Read the model definition and answer for the solid it produces. Units are mm, in the model's axes. A direction names the side the tool comes from. Coordinates: 2 decimals unless noted, no trailing zeros. Loops run counter-clockwise (first coordinate to the right, second up) from the corner with the lowest first, then second, coordinate; pieces in that order, holes last. Notation, with made-up numbers: M -34.75,-32 L -11.75,-32 A20 cw -11.75,-23 Z; hole C 37.5,-16.5 d10. An arc over 180 degrees is marked long. One line per item, written item: value. Start each with the question number.
1. Flat-ended cylindrical pins translate along their axes: pin 1 (15 mm diameter, centred on x = 52, z = 40, fed in from -Y); pin 2 (6 mm diameter, centred on x = 92.5, y = -17.5, fed in from -Z); pin 3 (8 mm diameter, centred on x = 57, z = 69.5, fed in from -Y); pin 4 (3 mm diameter, centred on x = 95.5, z = 4, fed in from -Y). Find the tip coordinate at first contact, or state that the pin passes through.
2. Consider probe 1 along X at (y, z) = (12.5, -2.5) (3 decimals); probe 2 along Y at (x, z) = (59, 47.5); probe 3 along Z at (x, y) = (17, 52) (3 decimals). Determine where each line is inside the solid, lowest interval first.
3. The part is cut by section A-A (y = -46). Write down the section's boundary in (x, z) (3 decimals), then the cut area to 3 significant figures.
4. The part is cut by section B-B (z = 110). Write down the section's boundary in (x, y).
5. For faces 1 (the face through (-2, 8.001, 31)), 2 (the face through (60, 0, 61.925)), 3 (the face through (109.2, -9.7, 52.6)), 4 (the face through (101, 10, 38.1)), determine the directions among +Z, -Z, +X, -X, +Y, -Y from which every point of the face is accessible in a straight line to the end or side of a thin tool.
```python
from build123d import *

# Parameters (mm, degrees)
F2_DEPTH     = 63.5
F0_W         = 25.4
F0_H         = 19.05
F3_DEPTH     = 25.4
F4_DEPTH     = 8.001
F6_R         = 6.35
F7_T1_DEPTH  = 17.4752
F7_T4_ANGLE  = 90
F7_T8_DEPTH  = 42.06875
F7_S9_R      = 25.4
F7_T10_DEPTH = 23
F7_T12_ANGLE = 90
F7_T14_ANGLE = 90
F7_T18_DEPTH = 42.06875
F7_S19_R     = 25.4
F7_T20_DEPTH = 23
F7_T22_ANGLE = 90
F7_T26_DEPTH = 42.06875
F7_S27_R     = 25.4
F7_T28_DEPTH = 23
F7_T32_DEPTH = 42.06875
F7_S33_R     = 25.4
F7_T34_DEPTH = 23
F8_R         = 19.05
F9_DEPTH     = 127


# Not quite as in the source:
# - a fillet or chamfer that OpenCascade refuses, or shapes differently, is made with other operations: its cross-section is extruded or revolved along the edge and cut away or added


with BuildPart() as f2:
    # F0 (on Front) → F2 (new body, symmetric)
    with BuildSketch(Plane.XZ):
        Polygon((22.225, 9.525), (-41.275, 9.525), (-41.275, -9.525), (41.275, -9.525), (41.275, 9.525), align=None)
    extrude(amount=F2_DEPTH, both=True)

    # F0 (on Front) → F3 (join, symmetric)
    with BuildSketch(Plane.XZ):
        with BuildLine():
            Line((22.225, 27.0002), (22.225, 9.525))
            Line((22.225, 9.525), (41.275, 9.525))
            Line((41.275, 9.525), (41.275, 27.0002))
            ThreePointArc((41.275, 27.0002), (45.9246798487, 38.2255201513), (57.15, 42.8752))
            Line((57.15, 42.8752), (60.325, 42.8752))
            Line((60.325, 42.8752), (60.325, 61.9252))
            Line((60.325, 61.9252), (57.15, 61.9252))
            ThreePointArc((57.15, 61.9252), (32.4542956671, 51.6959043329), (22.225, 27.0002))
        make_face()
        with Locations((73.025, 52.4002)):
            Rectangle(F0_W, F0_H)
    extrude(amount=F3_DEPTH, both=True)

    # F0 (on Front) → F4 (join, symmetric)
    with BuildSketch(Plane.XZ):
        with BuildLine():
            add(Edge.make_bspline(
                [(-41.275, 9.525), (-25.3429859877, 49.4523830712), (4.4616423547, 62.58662045), (57.15, 61.9252)],
                knots=[0, 0, 0, 0, 111.5045361635, 111.5045361635, 111.5045361635, 111.5045361635], degree=3))
            Line((-41.275, 9.525), (22.225, 9.525))
            Line((22.225, 9.525), (22.225, 27.0002))
            ThreePointArc((22.225, 27.0002), (32.4542956671, 51.6959043329), (57.15, 61.9252))
        make_face()
    extrude(amount=F4_DEPTH, both=True)

    # F0 (on Front) → F5 (revolve)
    with BuildSketch(Plane.XZ):
        Polygon((85.725, 66.675), (85.725, 61.9252), (85.725, 42.8752), (85.725, 38.1), (111.125, 38.1), (111.125, 66.675), align=None)
    revolve(axis=Axis((85.725, 0, 52.3875), (0, 0, 1)))

    # F6
    f6_edges = [f2.edges().sort_by_distance(p)[0] for p in [
        (41.275, -63.5, 0),
        (-41.275, -63.5, 0),
        (41.275, 63.5, 0),
        (-41.275, 63.5, 0),
    ]]
    fillet(f6_edges, radius=F6_R)

    # F7: fillet of radius 3.175 on 12 edges, made by hand

    # F7_s2 → F7_t1 (cut)
    with BuildSketch(Plane.XY.offset(9.525)):
        with BuildLine():
            ThreePointArc((25.4, -25.4), (23.1549359697, -24.4700640303), (22.225, -22.225))
            Line((22.225, -22.225), (22.225, -25.4))
            Line((22.225, -25.4), (25.4, -25.4))
        make_face()
        with BuildLine():
            ThreePointArc((41.275, -22.225), (40.3450640303, -24.4700640303), (38.1, -25.4))
            Line((38.1, -25.4), (41.275, -25.4))
            Line((41.275, -25.4), (41.275, -22.225))
        make_face()
        with BuildLine():
            ThreePointArc((25.4, 25.4), (23.1549359697, 24.4700640303), (22.225, 22.225))
            Line((22.225, 22.225), (22.225, 25.4))
            Line((22.225, 25.4), (25.4, 25.4))
        make_face()
        with BuildLine():
            ThreePointArc((41.275, 22.225), (40.3450640303, 24.4700640303), (38.1, 25.4))
            Line((38.1, 25.4), (41.275, 25.4))
            Line((41.275, 25.4), (41.275, 22.225))
        make_face()
    extrude(amount=F7_T1_DEPTH, mode=Mode.SUBTRACT)

    # F7_s3 → F7_t4 (revolve, cut)
    with BuildSketch(Plane.YZ.offset(57.15)):
        with BuildLine():
            ThreePointArc((-25.4, 58.7502), (-24.4700640303, 60.9952640303), (-22.225, 61.9252))
            Line((-22.225, 61.9252), (-25.4, 61.9252))
            Line((-25.4, 61.9252), (-25.4, 58.7502))
        make_face()
    revolve(axis=Axis((57.15, -25.4, 27.0002), (0, -1, 0)), revolution_arc=F7_T4_ANGLE, mode=Mode.SUBTRACT)


with BuildPart() as f7_tool6:
    # F7_s7 → F7_t8 (new body)
    with BuildSketch(Plane.YZ.offset(99.21875)):
        with BuildLine():
            ThreePointArc((-25.4, 58.7502), (-24.4700640303, 60.9952640303), (-22.225, 61.9252))
            Line((-22.225, 61.9252), (-25.4, 61.9252))
            Line((-25.4, 61.9252), (-25.4, 58.7502))
        make_face()
    extrude(amount=-F7_T8_DEPTH)

    # F7_s9 → F7_t10 (cut, symmetric)
    with BuildSketch(Plane.XY.offset(60.3)):
        with Locations((85.725, 0)):
            Circle(F7_S9_R)
    extrude(amount=F7_T10_DEPTH, both=True, mode=Mode.SUBTRACT)


with BuildPart() as f2_1:
    add(f2.part)

    # F7_t5: cut F7_tool6
    add(f7_tool6.part, mode=Mode.SUBTRACT)

    # F7_s11 → F7_t12 (revolve, cut)
    with BuildSketch(Plane.XY.offset(27.0002)):
        with BuildLine():
            ThreePointArc((41.275, -22.225), (40.3450640303, -24.4700640303), (38.1, -25.4))
            Line((38.1, -25.4), (41.275, -25.4))
            Line((41.275, -25.4), (41.275, -22.225))
        make_face()
    revolve(axis=Axis((57.15, -25.4, 27.0002), (0, 1, 0)), revolution_arc=F7_T12_ANGLE, mode=Mode.SUBTRACT)

    # F7_s13 → F7_t14 (revolve, cut)
    with BuildSketch(Plane.YZ.offset(57.15)):
        with BuildLine():
            ThreePointArc((25.4, 58.7502), (24.4700640303, 60.9952640303), (22.225, 61.9252))
            Line((22.225, 61.9252), (25.4, 61.9252))
            Line((25.4, 61.9252), (25.4, 58.7502))
        make_face()
    revolve(axis=Axis((57.15, 25.4, 27.0002), (0, -1, 0)), revolution_arc=F7_T14_ANGLE, mode=Mode.SUBTRACT)


with BuildPart() as f7_tool16:
    # F7_s17 → F7_t18 (new body)
    with BuildSketch(Plane.YZ.offset(99.21875)):
        with BuildLine():
            ThreePointArc((25.4, 58.7502), (24.4700640303, 60.9952640303), (22.225, 61.9252))
            Line((22.225, 61.9252), (25.4, 61.9252))
            Line((25.4, 61.9252), (25.4, 58.7502))
        make_face()
    extrude(amount=-F7_T18_DEPTH)

    # F7_s19 → F7_t20 (cut, symmetric)
    with BuildSketch(Plane.XY.offset(60.3)):
        with Locations((85.725, 0)):
            Circle(F7_S19_R)
    extrude(amount=F7_T20_DEPTH, both=True, mode=Mode.SUBTRACT)


with BuildPart() as f2_2:
    add(f2_1.part)

    # F7_t15: cut F7_tool16
    add(f7_tool16.part, mode=Mode.SUBTRACT)

    # F7_s21 → F7_t22 (revolve, cut)
    with BuildSketch(Plane.XY.offset(27.0002)):
        with BuildLine():
            ThreePointArc((38.1, 25.4), (40.3450640303, 24.4700640303), (41.275, 22.225))
            Line((41.275, 22.225), (41.275, 25.4))
            Line((41.275, 25.4), (38.1, 25.4))
        make_face()
    revolve(axis=Axis((57.15, 25.4, 27.0002), (0, 1, 0)), revolution_arc=F7_T22_ANGLE, mode=Mode.SUBTRACT)


with BuildPart() as f7_tool24:
    # F7_s25 → F7_t26 (new body)
    with BuildSketch(Plane.YZ.offset(57.15)):
        with BuildLine():
            ThreePointArc((25.4, 46.0502), (24.4700640303, 43.8051359697), (22.225, 42.8752))
            Line((22.225, 42.8752), (25.4, 42.8752))
            Line((25.4, 42.8752), (25.4, 46.0502))
        make_face()
    extrude(amount=F7_T26_DEPTH)

    # F7_s27 → F7_t28 (cut, symmetric)
    with BuildSketch(Plane.XY.offset(44.5)):
        with Locations((85.725, 0)):
            Circle(F7_S27_R)
    extrude(amount=F7_T28_DEPTH, both=True, mode=Mode.SUBTRACT)


with BuildPart() as f2_3:
    add(f2_2.part)

    # F7_t23: cut F7_tool24
    add(f7_tool24.part, mode=Mode.SUBTRACT)


with BuildPart() as f7_tool30:
    # F7_s31 → F7_t32 (new body)
    with BuildSketch(Plane.YZ.offset(57.15)):
        with BuildLine():
            ThreePointArc((-25.4, 46.0502), (-24.4700640303, 43.8051359697), (-22.225, 42.8752))
            Line((-22.225, 42.8752), (-25.4, 42.8752))
            Line((-25.4, 42.8752), (-25.4, 46.0502))
        make_face()
    extrude(amount=F7_T32_DEPTH)

    # F7_s33 → F7_t34 (cut, symmetric)
    with BuildSketch(Plane.XY.offset(44.5)):
        with Locations((85.725, 0)):
            Circle(F7_S33_R)
    extrude(amount=F7_T34_DEPTH, both=True, mode=Mode.SUBTRACT)


with BuildPart() as f2_4:
    add(f2_3.part)

    # F7_t29: cut F7_tool30
    add(f7_tool30.part, mode=Mode.SUBTRACT)

    # F8 (on Top) → F9 (join)
    with BuildSketch(Plane.XY):
        with Locations((84.2625681776, 0)):
            Circle(F8_R)
    extrude(amount=F9_DEPTH)


solid = f2_4.part
```
Answer block:
1. pin 1: stops at y = -25.4
1. pin 2: stops at z = 0
1. pin 3: passes through
1. pin 4: stops at y = -16.37
2. probe 1: x = -41.275 to 41.275
2. probe 2: y = -25.4 to 25.4
2. probe 3: z = -9.525 to 9.525
3. outline: M -41.275,-9.525 L 41.275,-9.525 L 41.275,9.525 L -41.275,9.525 Z
3. area: 1,570 mm2
4. outline: C 84.26,0 d38.1
5. face 1: +Z, -X, +Y
5. face 2: +Z, -X
5. face 3: none
5. face 4: -Z
